Here's how the part is built. I have some questions about the finished solid (model axes, mm). Coordinates: 2 decimals unless noted, no trailing zeros. Order: outer loops, then holes, each group sorted by start corner. A loop starts at its lowest first (then second) coordinate and runs counter-clockwise, first axis right, second up. Notation, with made-up numbers: (84.25, -9.5) -> (138.25, -9.5) arc R22 cw to (138.25, 25.5) -> close; hole circle Ø7 at (75.25, 43). An arc over 180 degrees is marked (long way). One line per item, written item: value. Start each with the question number.
```python
from build123d import *

# Parameters (mm, degrees)
SKETCH_1_W          = 12
SKETCH_1_H          = 50
EXTRUDE_1_DEPTH     = 5
SKETCH_2_R          = 1.5
CUT_EXTRUDE_1_DEPTH = 27.191601707
FILLET_2_R          = 3


with BuildPart() as part:
    # 草图1 → 凸台-拉伸1 (new body)
    with BuildSketch(Plane.XY):
        Rectangle(SKETCH_1_W, SKETCH_1_H)
    extrude(amount=EXTRUDE_1_DEPTH)

    # 草图2 → 切除-拉伸1 (cut, through all)
    with BuildSketch(Plane.XY.offset(5)):
        with Locations((0, 15)):
            Circle(SKETCH_2_R)
    cut_extrude_1 = extrude(amount=-CUT_EXTRUDE_1_DEPTH, mode=Mode.SUBTRACT)

    # 镜向1: 切除-拉伸1 across plane
    add(cut_extrude_1.mirror(Plane.ZX), mode=Mode.SUBTRACT)

    # 圆角2
    fillet_2_edges = [part.edges().sort_by_distance(p)[0] for p in [
        (-6, 25, 2.5),
    ]]
    fillet(fillet_2_edges, radius=FILLET_2_R)


solid = part.part
```
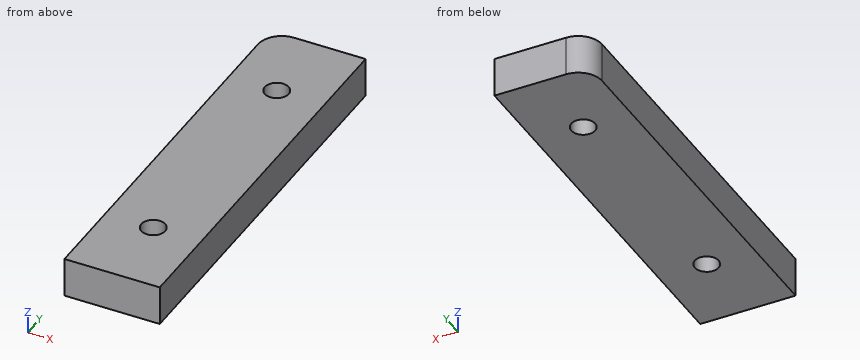
Q1. Imagine slicing it at A-A (y = 15). Write out the boundary of the cut face in (x, z), plus the area to 3 significant figures.
Q2. I need wall thicknesses on line 1 (Y direction, x = 0, z = 2.75); line 2 (X direction, y = -15, z = 3.4); line 3 (Y direction, x = -0.75, z = 0.9). Which ranges of each line are inside material? Lowest first, please.
Q3. Imagine slicing it at D-D (y = -14). Write out the boundary of the cut face in (x, z), plus the area to 3 significant figures.
Q4. Imagine slicing it at C-C (x = 0). Write out the boundary of the cut face in (y, z), plus the area to 3 significant figures.
Q5. Imagine slicing it at B-B (z = 3.6). Write out the boundary of the cut face in (x, y).
Completed:
1. outline: (-6, 0) -> (-1.5, 0) -> (-1.5, 5) -> (-6, 5) -> close; (1.5, 0) -> (6, 0) -> (6, 5) -> (1.5, 5) -> close
1. area: 45.0 mm2
2. line 1: y = -25 to -16.5, -13.5 to 13.5, 16.5 to 25
2. line 2: x = -6 to -1.5, 1.5 to 6
2. line 3: y = -25 to -16.3, -13.7 to 13.7, 16.3 to 25
3. outline: (-6, 0) -> (-1.12, 0) -> (-1.12, 5) -> (-6, 5) -> close; (1.12, 0) -> (6, 0) -> (6, 5) -> (1.12, 5) -> close
3. area: 48.8 mm2
4. outline: (-25, 0) -> (-16.5, 0) -> (-16.5, 5) -> (-25, 5) -> close; (-13.5, 0) -> (13.5, 0) -> (13.5, 5) -> (-13.5, 5) -> close; (16.5, 0) -> (25, 0) -> (25, 5) -> (16.5, 5) -> close
4. area: 220 mm2
5. outline: (-6, -25) -> (6, -25) -> (6, 25) -> (-3, 25) arc R3 ccw to (-6, 22) -> close; hole circle Ø3 at (0, -15); hole circle Ø3 at (0, 15)
